Source: CAD feature listing. Evaluate the final solid. Frame: model axes, mm. Coordinates: 2 decimals unless noted, no trailing zeros. Loops run counter-clockwise (first coordinate to the right, second up) from the corner with the lowest first, then second, coordinate; pieces in that order, holes last. Notation, with made-up numbers: (62, -31.75) -> (69, -31.75) arc R9 ccw to (69, -15.75) -> close; hole circle Ø7 at (-6, -7). An arc over 180 degrees is marked (long way). Answer as a JSON object with one key per item and string values. Group by question number.
from build123d import *

# Parameters (mm, degrees)
F1_DEPTH = 25.4


with BuildPart() as f1:
    # F0 (on Top) → F1 (new body)
    with BuildSketch(Plane.XY):
        with BuildLine():
            Line((17.489951, 31.716853), (-26.626494, 31.716853))
            Line((-26.626494, 31.716853), (-26.626494, -54.166641))
            ThreePointArc((-26.626494, -54.166641), (-24.574217, -63.510594), (-18.795172, -71.1345))
            ThreePointArc((-18.795172, -71.1345), (-8.568909, -76.317285), (2.871485, -75.572252))
            ThreePointArc((2.871485, -75.572252), (13.486649, -67.127156), (17.489951, -54.166641))
            Line((17.489951, -54.166641), (17.489951, 31.716853))
        make_face()
    extrude(amount=F1_DEPTH)


solid = f1.part
1. Section query B-B on x = 4. Return loops of the section in (y, z), then the cut area to 3 significant figures.
2. Ray query, L1, parallel to X at y = -69.5, z = 22.5; L2, parallel to Y at x = -8, z = 7.25; L3, parallel to Y at x = -19, z = 23.5. Return the intervals inside material, ascending.
3. Section query A-A on z = 8.75. Return loops of the section in (x, y) (1 decimal), then the cut area to 3 significant figures.
4. Pin query (flat end, axial travel): pin 1 Ø5 at (x, z) = (1, 19) entering from -Y. Return the tip coordinate at first contact, or that it passes through.
5. Section query C-C on x = -14.5. Return loops of the section in (y, z).
Solved:
{
 "1": {"outline": "(-75.1, 0) -> (31.72, 0) -> (31.72, 25.4) -> (-75.1, 25.4) -> close", "area": "2,710 mm^2"},
 "2": {"L1": "-20.52 to 11.63", "L2": "-76.43 to 31.72", "L3": "-70.96 to 31.72"},
 "3": {"outline": "(-26.6, -54.2) arc R22.3 ccw to (-18.8, -71.1) arc R21.7 ccw to (2.9, -75.6) arc R23 ccw to (17.5, -54.2) -> (17.5, 31.7) -> (-26.6, 31.7) -> close", "area": "4,570 mm^2"},
 "4": {"pin 1": "y = -76.59"},
 "5": {"outline": "(-74.17, 0) -> (31.72, 0) -> (31.72, 25.4) -> (-74.17, 25.4) -> close"}
}
